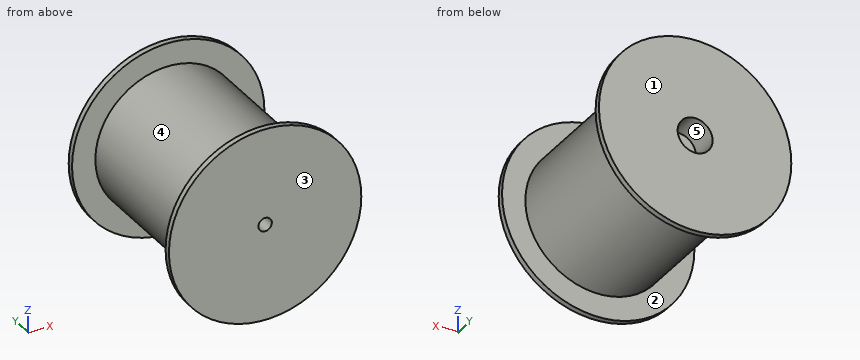
from build123d import *

# Parameters (mm, degrees)
ESQUISSE1_R             = 12.5
BOSS_EXTRU_1_DEPTH      = 30
ESQUISSE1_3_R           = 16.5
ESQUISSE1_3_R_2         = 12.5
BOSS_EXTRU_2_DEPTH      = 1
ESQUISSE2_R             = 16.5
BOSS_EXTRU_3_DEPTH      = 1
ESQUISSE3_R             = 1.1525
ENL_V_MAT_EXTRU_1_DEPTH = 6
ESQUISSE4_R             = 3
ENL_V_MAT_EXTRU_2_DEPTH = 5


with BuildPart() as part:
    # Esquisse1 → Boss.-Extru.1 (new body)
    with BuildSketch(Plane(origin=(0, 0, 0), x_dir=(1, 0, 0), z_dir=(0, 1, 0))):
        Circle(ESQUISSE1_R)
    extrude(amount=BOSS_EXTRU_1_DEPTH)

    # Esquisse1_3 → Boss.-Extru.2 (add)
    with BuildSketch(Plane(origin=(0, 0, 0), x_dir=(1, 0, 0), z_dir=(0, 1, 0))):
        Circle(ESQUISSE1_3_R)
        Circle(ESQUISSE1_3_R_2, mode=Mode.SUBTRACT)
    extrude(amount=BOSS_EXTRU_2_DEPTH)

    # Esquisse2 → Boss.-Extru.3 (add)
    with BuildSketch(Plane(origin=(0, 30, 0), x_dir=(1, 0, 0), z_dir=(0, 1, 0))):
        Circle(ESQUISSE2_R)
    extrude(amount=-BOSS_EXTRU_3_DEPTH)

    # Esquisse3 → Enl_v. mat.-Extru.1 (cut)
    with BuildSketch(Plane.XZ):
        Circle(ESQUISSE3_R)
    extrude(amount=-ENL_V_MAT_EXTRU_1_DEPTH, mode=Mode.SUBTRACT)

    # Esquisse4 → Enl_v. mat.-Extru.2 (cut)
    with BuildSketch(Plane(origin=(0, 30, 0), x_dir=(1, 0, 0), z_dir=(0, 1, 0))):
        Circle(ESQUISSE4_R)
    extrude(amount=-ENL_V_MAT_EXTRU_2_DEPTH, mode=Mode.SUBTRACT)


solid = part.part
Verification items for the finished model (mm, model axes). Face numbers are marked on the shaded views. A direction names the side the tool comes from. Round coordinates to 2 decimals unless told otherwise and drop trailing zeros. Write each loop counter-clockwise with the first axis right and the second up, starting at its lowest first coordinate (ties: lowest second). Pieces come first, ordered by that corner, then holes.
(1) Section check C-C (y = 2). Enter the section's corners in (x, z) (1 decimal).
Returned:
outline: circle Ø25 at (0, 0); hole circle Ø2.3 at (0, 0)
(2) Section check D-D (z = 0). Enter the section's corners in (x, y), plus the area to 3 significant figures.
Returned:
outline: (-16.5, 0) - (-1.15, 0) - (-1.15, 6) - (1.15, 6) - (1.15, 0) - (16.5, 0) - (16.5, 1) - (12.5, 1) - (12.5, 29) - (16.5, 29) - (16.5, 30) - (3, 30) - (3, 25) - (-3, 25) - (-3, 30) - (-16.5, 30) - (-16.5, 29) - (-12.5, 29) - (-12.5, 1) - (-16.5, 1) - close
area: 722 mm2
(3) Depth check by flat-ended pin: pin 1 Ø12 at (y, z) = (16, 9.5) entering from -X; pin 2 Ø12 at (x, y) = (1.5, 10.5) entering from +Z; pin 3 Ø1.2 at (x, z) = (0.5, 0) entering from -Y; pin 4 Ø5 at (x, z) = (1, -0.5) entering from +Y. Enter the tip coordinate at first touch or a pass-through.
Returned:
pin 1: stops at x = -12
pin 2: stops at z = 12.5
pin 3: stops at y = 6
pin 4: stops at y = 30
(4) Section check B-B (z = -13). Enter the section's corners in (x, y), plus the area to 3 significant figures.
Returned:
outline: (-10.16, 0) - (10.16, 0) - (10.16, 1) - (-10.16, 1) - close; (-10.16, 29) - (10.16, 29) - (10.16, 30) - (-10.16, 30) - close
area: 40.6 mm2
(5) Access from +Z, -Z, +X, -X, +Y, -Y to the whole of each face (thin tool, end or side, straight path). Record for the marked faces 4 and 5.
Returned:
face 4: none
face 5: +Y
(6) Mould release check, pull along Y, two halves, no side actions. Record for the marked faces 1, 2 and 3: pulls with the +Y half, pulls with the -Y half, needs draft (parallel to the pull), parting line crosses it, or undercut.
Returned:
face 1: pulls with the +Y half
face 2: undercut
face 3: pulls with the -Y half
(7) Section check A-A (x = 0). Enter the section's corners in (y, z).
Returned:
outline: (0, -16.5) - (1, -16.5) - (1, -12.5) - (29, -12.5) - (29, -16.5) - (30, -16.5) - (30, -3) - (25, -3) - (25, 3) - (30, 3) - (30, 16.5) - (29, 16.5) - (29, 12.5) - (1, 12.5) - (1, 16.5) - (0, 16.5) - (0, 1.15) - (6, 1.15) - (6, -1.15) - (0, -1.15) - close
(8) Material ranges on line 1 (Z direction, x = 0, y = 26.7); line 2 (Y direction, x = 8.5, z = 11.5), recorded low to high.
Returned:
line 1: z = -12.5 to -3, 3 to 12.5
line 2: y = 0 to 1, 29 to 30
